from build123d import *

# Parameters (mm, degrees)
ESQUISSE1_R             = 29
BOSS_EXTRU_1_DEPTH      = 30
ESQUISSE2_R             = 4
BOSS_EXTRU_2_DEPTH      = 6
ESQUISSE3_R             = 5
BOSS_EXTRU_3_DEPTH      = 2
ESQUISSE4_R             = 4
ENL_V_MAT_EXTRU_1_DEPTH = 5
CHANFREIN1_SIZE         = 1
ESQUISSE5_R             = 4
BOSS_EXTRU_4_DEPTH      = 10
ESQUISSE6_R             = 4
BOSS_EXTRU_5_DEPTH      = 28
CHANFREIN2_SIZE         = 1


with BuildPart() as part:
    # Esquisse1 → Boss.-Extru.1 (new body)
    with BuildSketch(Plane.XY):
        Circle(ESQUISSE1_R)
    extrude(amount=BOSS_EXTRU_1_DEPTH)

    # Esquisse2 → Boss.-Extru.2 (add)
    with BuildSketch(Plane.XY.offset(30)):
        Circle(ESQUISSE2_R)
    extrude(amount=BOSS_EXTRU_2_DEPTH)

    # Esquisse3 → Boss.-Extru.3 (add)
    with BuildSketch(Plane.XY.offset(30)):
        Circle(ESQUISSE3_R)
    extrude(amount=BOSS_EXTRU_3_DEPTH)

    # Esquisse4 → Enlèv. mat.-Extru.1 (cut)
    with BuildSketch(Plane(origin=(0, 0, 0), x_dir=(-1, 0, 0), z_dir=(0, 0, -1))):
        with Locations(Location((0, 0, 0), (0, 0, 180))):
            Circle(ESQUISSE4_R)
    extrude(amount=-ENL_V_MAT_EXTRU_1_DEPTH, mode=Mode.SUBTRACT)

    # Chanfrein1
    chanfrein1_edges = [part.edges().sort_by_distance(p)[0] for p in [
        (-29, 0, 0),
        (-29, 0, 30),
    ]]
    chamfer(chanfrein1_edges, length=CHANFREIN1_SIZE)

    # Esquisse5 → Boss.-Extru.4 (add)
    with BuildSketch(Plane.XY.offset(36)):
        Circle(ESQUISSE5_R)
    extrude(amount=BOSS_EXTRU_4_DEPTH)

    # Esquisse6 → Boss.-Extru.5 (add)
    with BuildSketch(Plane.XY.offset(46)):
        Circle(ESQUISSE6_R)
    extrude(amount=BOSS_EXTRU_5_DEPTH)

    # Chanfrein2
    chanfrein2_edges = [part.edges().sort_by_distance(p)[0] for p in [
        (-4, 0, 74),
    ]]
    chamfer(chanfrein2_edges, length=CHANFREIN2_SIZE)


solid = part.part
Part model, mm, in its own coordinate system. A direction names the side the tool comes from. Round coordinates to 2 decimals unless told otherwise and drop trailing zeros. Loops run counter-clockwise (first coordinate to the right, second up) from the corner with the lowest first, then second, coordinate; pieces in that order, holes last. Notation, with made-up numbers: (11, -29.75) - (38, -29.75) arc R17 cw to (38, -2.75) - close; hole circle Ø11 at (47.25, 52). An arc over 180 degrees is marked (long way). Answer as a JSON object with one key per item and string values.
Item 1: Pull direction X, two halves, no side cores. Call faces 1 (the face through (-1.08, -4.88, 30.99)), 2 (the face through (0, 0, 74)), 3 (the face through (-0.867, 3.905, 2.465)): pulls with the +X half, pulls with the -X half, needs draft (parallel to the pull), parting line crosses it, or undercut.
Output:
{"face 1": "parting line crosses it", "face 2": "needs draft", "face 3": "undercut"}
Item 2: Band-saw the part on C-C on z = 28. List the corners of the cut face in (x, y), plus the area to 3 significant figures.
Output:
{"outline": "circle Ø58 at (0, 0)", "area": "2,640 mm2"}
Item 3: Pin check, flat tips, straight feed: pin 1 (3 mm diameter, centred on y = -20, z = 24.5, fed in from +X); pin 2 (10 mm diameter, centred on x = -2.5, z = 27.5, fed in from +Y). Stop position of each tip, or through.
Output:
{"pin 1": "x = 22.33", "pin 2": "y = 29"}
Item 4: Tool access for faces 4 (the face through (-0.867, -3.905, 52.213)), 5 (the face through (13.38, -25.73, 14.8)), 6 (the face through (0, 0, 5)): list every direction of +Z, -Z, +X, -X, +Y, -Y with a clear straight run to the whole face (end or side of a thin tool).
Output:
{"face 4": "+Z", "face 5": "+Z, -Z", "face 6": "-Z"}
Item 5: Wall check: L1, parallel to Y at x = 0, z = 1.15; L2, parallel to Z at x = -17, y = -18; L3, parallel to X at y = 0, z = 45. Give the ranges that are in metal, low to high.
Output:
{"L1": "-29 to -4, 4 to 29", "L2": "0 to 30", "L3": "-4 to 4"}
Item 6: Band-saw the part on A-A on x = 0. List the corners of the cut face in (y, z).
Output:
{"outline": "(-29, 1) - (-28, 0) - (-4, 0) - (-4, 5) - (4, 5) - (4, 0) - (28, 0) - (29, 1) - (29, 29) - (28, 30) - (5, 30) - (5, 32) - (4, 32) - (4, 73) - (3, 74) - (-3, 74) - (-4, 73) - (-4, 32) - (-5, 32) - (-5, 30) - (-28, 30) - (-29, 29) - close"}
